from build123d import *

# Parameters (mm, degrees)
F0_W          = 75
F0_H          = 72.5740331761
F1_DEPTH      = 50
F1_DEPTH_BACK = 50


with BuildPart() as f1:
    # F0 (on Front) → F1 (new body, two sides)
    with BuildSketch(Plane.XZ) as f1_sk:
        Polygon((-34.9110340909, 68.1764709135), (-55.4926691404, 48.7848244566), (-55.4926691404, -26.2151755434), (-34.9110340909, -48.9259438893), (40.0889659091, -48.9259438893), (62.090027551, -26.2151755434), (62.090027551, 48.7848244566), (40.0889659091, 68.1764709135), align=None)
        with Locations((2.5889659091, 12.4978078685)):
            Rectangle(F0_W, F0_H, mode=Mode.SUBTRACT)
    extrude(amount=-F1_DEPTH)
    extrude(f1_sk.sketch, amount=F1_DEPTH_BACK)


solid = f1.part
CAD build for the part. Positions are in the model's coordinates, mm. A direction names the side the tool comes from. Round coordinates to 2 decimals unless told otherwise and drop trailing zeros. Loops run counter-clockwise (first coordinate to the right, second up) from the corner with the lowest first, then second, coordinate; pieces in that order, holes last. Notation, with made-up numbers: (32, 78.25) - (64, 78.25) arc R23 cw to (64, 91.25) - close; hole circle Ø10 at (78.5, 18.25). An arc over 180 degrees is marked (long way). Put each result on its own line as item: value.
1. Slice it at A-A on x = -20. List the corners of the cut face in (y, z), and give its area (3 significant figures).
Geometry check:
outline: (-50, -48.93) - (50, -48.93) - (50, -23.79) - (-50, -23.79) - close; (-50, 48.78) - (50, 48.78) - (50, 68.18) - (-50, 68.18) - close
area: 4,450 mm²
2. Slice it at D-D on x = -39. List the corners of the cut face in (y, z).
Geometry check:
outline: (-50, -44.41) - (50, -44.41) - (50, 64.32) - (-50, 64.32) - close
3. Wall check: line 1 (X direction, y = 24.5, z = 9); line 2 (Z direction, x = -20, y = -14); line 3 (Z direction, x = -44, y = -19). Give the ranges that are in metal, low to high.
Geometry check:
line 1: -55.49 to -34.91, 40.09 to 62.09
line 2: -48.93 to -23.79, 48.78 to 68.18
line 3: -38.9 to 59.61
4. Slice it at C-C on z = 21.5. List the corners of the cut face in (x, y), and give its area (3 significant figures).
Geometry check:
outline: (-55.49, -50) - (-34.91, -50) - (-34.91, 50) - (-55.49, 50) - close; (40.09, -50) - (62.09, -50) - (62.09, 50) - (40.09, 50) - close
area: 4,260 mm²
5. Two-plate mould, pull along X, no slides. Class faces 3 (the flat face through (2, -50, 49)), 4 (the flat face through (2, 1, 48.785)), 5 (the flat face through (-45.35, 0.7, -37.41)), 6 (the flat face through (40.089, 1, 12)): released by +X, released by -X, zero draft, split by the parting line, or undercut.
Geometry check:
face 3: zero draft
face 4: undercut
face 5: released by -X
face 6: undercut
6. Slice it at B-B on y = 17. List the corners of the cut face in (x, z), and give its area (3 significant figures).
Geometry check:
outline: (-55.49, -26.22) - (-34.91, -48.93) - (40.09, -48.93) - (62.09, -26.22) - (62.09, 48.78) - (40.09, 68.18) - (-34.91, 68.18) - (-55.49, 48.78) - close; hole (-34.91, -23.79) - (40.09, -23.79) - (40.09, 48.78) - (-34.91, 48.78) - close
area: 7,430 mm²
7. 3-axis set-ups, long thin cutter, end or side, ignore diameter. For faces 1 (the flat face through (2, 1, -48.926)), 2 (the flat face through (-34.911, 1, 12)): which of +Z, -Z, +X, -X, +Y, -Y reach the whole face in a straight line?
Geometry check:
face 1: -Z, +X, -X, +Y, -Y
face 2: +Y, -Y
